from build123d import *

# Parameters (mm, degrees)
F1_R     = 4.7625
F2_DEPTH = 6
F1_R_2   = 15.875
F1_R_3   = 1.5
F3_DEPTH = 3


with BuildPart() as f2:
    # F1 (on Top) → F2 (new body)
    with BuildSketch(Plane.XY):
        with Locations((33.2608025707, -165.5893599715)):
            Circle(F1_R)
        with BuildLine():
            ThreePointArc((35.2608025707, -167.3278938366), (33.2608025707, -168.2393599715), (31.2608025707, -167.3278938366))
            ThreePointArc((31.2608025707, -167.3278938366), (30.6132217472, -165.7025667882), (31.1196992314, -164.0278938366))
            ThreePointArc((31.1196992314, -164.0278938366), (33.2608025707, -162.9393599715), (35.4019059099, -164.0278938366))
            ThreePointArc((35.4019059099, -164.0278938366), (35.7803683913, -164.768209513), (35.9108025707, -165.5893599715))
            ThreePointArc((35.9108025707, -165.5893599715), (35.7429891068, -166.5173955312), (35.2608025707, -167.3278938366))
        make_face(mode=Mode.SUBTRACT)
        with BuildLine():
            ThreePointArc((35.4019059099, -164.0278938366), (33.2608025707, -162.9393599715), (31.1196992314, -164.0278938366))
            Line((31.1196992314, -164.0278938366), (35.4019059099, -164.0278938366))
        make_face()
        with BuildLine():
            Line((35.2608025707, -167.3278938366), (31.2608025707, -167.3278938366))
            ThreePointArc((31.2608025707, -167.3278938366), (33.2608025707, -168.2393599715), (35.2608025707, -167.3278938366))
        make_face()
    extrude(amount=F2_DEPTH)

    # F1 (on Top) → F3 (join)
    with BuildSketch(Plane.XY):
        with Locations((33.2608025707, -165.5893599715)):
            Circle(F1_R_2)
        with Locations((22.8684977253, -171.5893599715)):
            Circle(F1_R_3, mode=Mode.SUBTRACT)
        with Locations((43.6531074161, -171.5893599715)):
            Circle(F1_R_3, mode=Mode.SUBTRACT)
        with Locations((33.2608025707, -165.5893599715)):
            Circle(F1_R, mode=Mode.SUBTRACT)
        with Locations((33.2608025707, -153.5893599715)):
            Circle(F1_R_3, mode=Mode.SUBTRACT)
    extrude(amount=F3_DEPTH)


solid = f2.part
The listing builds one solid part. Answer for the finished solid, in the listing's coordinates (mm). A direction names the side the tool comes from. Round coordinates to 2 decimals unless told otherwise and drop trailing zeros. Order: outer loops, then holes, each group sorted by start corner. A loop starts at its lowest first (then second) coordinate and runs counter-clockwise, first axis right, second up. Notation, with made-up numbers: (0, -19.75) -> (6, -19.75) arc R8 cw to (6, -14.75) -> close; hole circle Ø5 at (-27, 47). An arc over 180 degrees is marked (long way). Put each result on its own line as item: value.
Q1. Determine the mould class of faces 4 (the cylindrical face through (30.614, -165.728, 2.958)), 5 (the flat face through (33, -168, 6)), 6 (the cylindrical face through (35.458, -169.815, 4.479)) for opening direction X: pulls with the +X half, pulls with the -X half, needs draft (parallel to the pull), parting line crosses it, or undercut.
Results list:
face 4: undercut
face 5: needs draft
face 6: parting line crosses it
Q2. Each of these flat-tipped pins is pushed along its axis until it touches: P1, Ø2.5, axis at x = 43.65, y = -171.59, coming from the -Z side (3 decimals); P2, Ø1.2, axis at x = 33.5, z = 4, coming from the +Y side; P3, Ø12, axis at x = 45.5, y = -155.5, coming from the +Z side; P4, Ø1.5, axis at x = 34.5, z = 5, coming from the -Y side. Where does it stop, or does it pass through?
Results list:
P1: through
P2: y = -160.83
P3: z = 3
P4: y = -170.33
Q3. Consider line 1 along Y through (x, z) = (32, 2.9); line 2 along Y through (x, z) = (33, 4.7); line 3 along Z through (x, y) = (21, -165). Determine where each line is inside the solid, lowest interval first.
Results list:
line 1: -181.41 to -167.33, -164.03 to -154.4, -152.78 to -149.76
line 2: -170.34 to -167.33, -164.03 to -160.83
line 3: 0 to 3
Q4. Section A-A, the plane x = 43.5 is taken. Write down the section's boundary in (y, z), and give its area (3 significant figures).
Results list:
outline: (-177.72, 0) -> (-173.08, 0) -> (-173.08, 3) -> (-177.72, 3) -> close; (-170.1, 0) -> (-153.46, 0) -> (-153.46, 3) -> (-170.1, 3) -> close
area: 63.8 mm^2
Q5. Section B-B, the plane y = -154.5 is taken. Write down the section's boundary in (x, z), and give its area (3 significant figures).
Results list:
outline: (21.9, 0) -> (32.07, 0) -> (32.07, 3) -> (21.9, 3) -> close; (34.45, 0) -> (44.62, 0) -> (44.62, 3) -> (34.45, 3) -> close
area: 61.0 mm^2
Q6. Which of the six approach directions +Z, -Z, +X, -X, +Y, -Y give full straight-line access (tool end or side, diameter ignored) to faces 1 (the flat face through (37, -165, 0)), 2 (the flat face through (37, -162, 3)), 3 (the flat face through (33, -164.028, 3))?
Results list:
face 1: -Z, +X, -X, +Y, -Y
face 2: +Z
face 3: +Z, -Z
Q7. Section C-C, the plane x = 34 is taken. Write down the section's boundary in (y, z), and give its area (3 significant figures).
Results list:
outline: (-181.45, 0) -> (-167.33, 0) -> (-167.33, 6) -> (-170.29, 6) -> (-170.29, 3) -> (-181.45, 3) -> close; (-164.03, 0) -> (-154.89, 0) -> (-154.89, 3) -> (-160.88, 3) -> (-160.88, 6) -> (-164.03, 6) -> close; (-152.28, 0) -> (-149.73, 0) -> (-149.73, 3) -> (-152.28, 3) -> close
area: 95.7 mm^2
